Here's the drawing with two shaded views (mm, measured from the low corner). I have some questions. A direction names the side the tool comes from. Give positions to 0.01 mm unless a question says otherwise; leave off trailing zeros. Loops run counter-clockwise (first coordinate to the right, second up) from the corner with the lowest first, then second, coordinate; pieces in that order, holes last. Notation, with made-up numbers: (-37.75, 61) - (-5.75, 61) arc R16 cw to (-5.75, 67) - close; hole circle Ø5 at (-7, 8.25). An arc over 180 degrees is marked (long way). Write each question's results on one line, items separated by ' | '. Start each with the question number.
1) I want a section at A-A, the plane y = 16. Write out the boundary of the cut face in (x, z), and give its area (3 significant figures).
2) I'm going to push flat-ended pins straight in: pin 1 (3 mm diameter, centred on x = 13, y = 5.5, fed in from +Z); pin 2 (4.5 mm diameter, centred on y = 8, z = 28, fed in from -X); pin 3 (3 mm diameter, centred on x = 29, y = 7, fed in from +Z); pin 4 (3 mm diameter, centred on y = 12.5, z = 10, fed in from +X). Where does each tip first touch, or does it pass through?
3) I want a section at C-C, the plane z = 28.5. Write out the boundary of the cut face in (x, y).
4) If I drill on probe 1 along Y at (x, z) = (29.5, 1.85); probe 2 along Y at (x, z) = (29.5, 0.85); probe 3 along Z at (x, y) = (1.6, 8), over which ranges is the centre line in solid material (lowest first)? Write a range as [from, to].
5) On a 3-axis mill with a long thin cutter (end or side, diameter ignored), from which of +Z, -Z, +X, -X, +Y, -Y can I reach the whole of each face in a straight line? I mean the marked faces 1 and 2. Say none if no direction works.
6) I want a section at B-B, the plane x = 14.5. Write out the boundary of the cut face in (y, z).
7) I want a section at D-D, the plane y = 2.5. Write out the boundary of the cut face in (x, z).
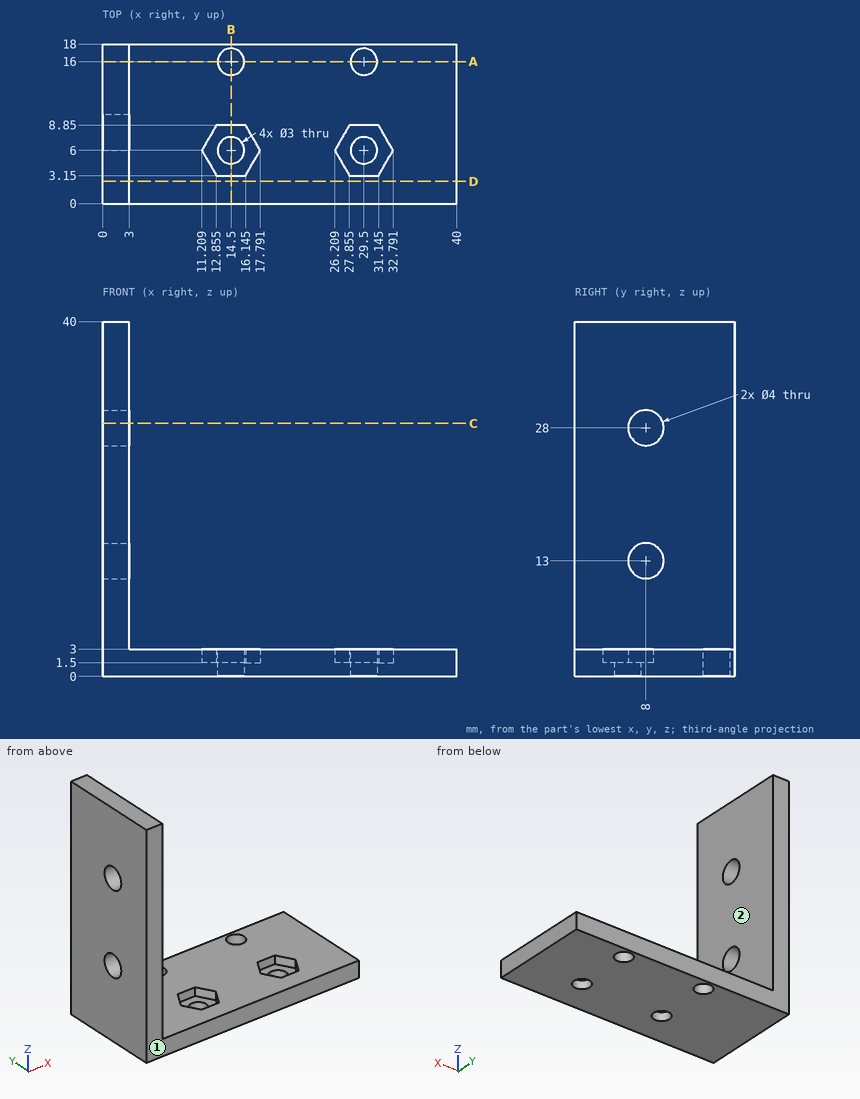
Answers:
1) outline: (0, 0) - (13, 0) - (13, 3) - (3, 3) - (3, 40) - (0, 40) - close; (16, 0) - (28, 0) - (28, 3) - (16, 3) - close; (31, 0) - (40, 0) - (40, 3) - (31, 3) - close | area: 213 mm2
2) pin 1: stops at z = 3 | pin 2: stops at x = 0 | pin 3: stops at z = 1.5 | pin 4: stops at x = 3
3) outline: (0, 0) - (3, 0) - (3, 6.06) - (0, 6.06) - close; (0, 9.94) - (3, 9.94) - (3, 18) - (0, 18) - close
4) probe 1: y = [0, 3.15], [8.85, 14.5], [17.5, 18] | probe 2: y = [0, 4.5], [7.5, 14.5], [17.5, 18] | probe 3: z = [0, 11], [15, 26], [30, 40]
5) face 1: +Z, -Z, +X, -X, -Y | face 2: +Z, +X, +Y, -Y
6) outline: (0, 0) - (4.5, 0) - (4.5, 1.5) - (3.15, 1.5) - (3.15, 3) - (0, 3) - close; (7.5, 0) - (14.5, 0) - (14.5, 3) - (8.85, 3) - (8.85, 1.5) - (7.5, 1.5) - close; (17.5, 0) - (18, 0) - (18, 3) - (17.5, 3) - close
7) outline: (0, 0) - (40, 0) - (40, 3) - (3, 3) - (3, 40) - (0, 40) - close
